Build history of the part. All positions in model axes, mm. Face numbers are marked on the shaded views. Give positions to 0.01 mm unless a question says otherwise; leave off trailing zeros. Loops run counter-clockwise (first coordinate to the right, second up) from the corner with the lowest first, then second, coordinate; pieces in that order, holes last. Notation, with made-up numbers: (15, -6.75) -> (32, -6.75) arc R24 ccw to (32, 20.25) -> close; hole circle Ø10 at (55.25, 40). An arc over 180 degrees is marked (long way). Answer as a JSON object with one key per item and string values. Group by question number.
Q1. Band-saw the part on C-C, the plane x = 7.5. Write the cut outline in (y, z).
Q2. Drop a flat-ended pin along its axis: pin 1 (1.5 mm diameter, centred on x = 18, z = 1, fed in from +Y). Give the stop position or say it passes through.
Q3. Band-saw the part on A-A, the plane y = 0. Write the cut outline in (x, z), plus the area to 3 significant figures.
Q4. Two-plate mould, pull along X, no slides. Class the marked faces 1 and 2: pulls with the +X half, pulls with the -X half, needs draft (parallel to the pull), parting line crosses it, or undercut.
Q5. Band-saw the part on D-D, the plane x = -8.5. Write the cut outline in (y, z).
Q6. Wall check: probe 1 along X at (y, z) = (1.55, -0.7); probe 2 along Y at (x, z) = (-23.5, 0.2); probe 3 along Y at (x, z) = (-2.5, 0.1). Give the ranges that are in metal, low to high. Write a range as from..to.
Autodesk Inventor part; units mm, degrees
ref_plane "YZ Plane" through (0, 0, 0) normal (1, 0, 0) x (0, 1, 0)
ref_plane "XZ Plane" through (0, 0, 0) normal (0, 1, 0) x (-1, 0, 0)
ref_plane "XY Plane" through (0, 0, 0) normal (0, 0, 1) x (1, 0, 0)
sketch "Sketch1" plane through (0, 0, 0) normal (0, 1, 0) x (-1, 0, 0)
  line L0 (13, 2) -> (13, 1.5)
  line L1 (13, 1.5) -> (0, 1.5)
  line L2 (28, 0) -> (28, 2)
  line L3 (28, 2) -> (13, 2)
  line L4 (0, 1.5) -> (0, 2)
  line L5 (0, 2) -> (-30, 2)
  line L6 (-30, 2) -> (-30, 0)
  line L7 (28, 0) -> (0, 0)
  line L8 (0, 0) -> (-30, 0)
  dimension "d5" = 0.5
  dimension "d6" = 15
  dimension "d7" = 0.5
  dimension "d8" = 2
  dimension "d9" = 28
  dimension "d10" = 30
  dimension "d12" = 4
revolve "Revolution1" add sketch "Sketch1" angle 360 about axis through (-28, 0, 0) along (1, 0, 0)
equation "\"d6\" = parA"
equation "\"d9\" = parH"
equation "\"d10\" = stroke"
properties part number "cylinderRod"
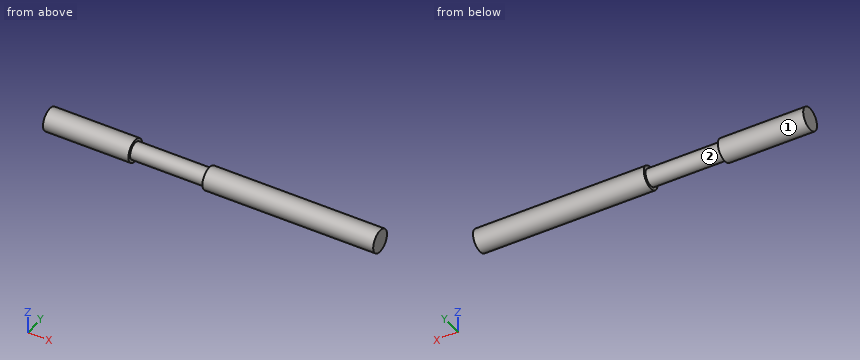
Worked answers:
{
 "1": {"outline": "circle Ø4 at (0, 0)"},
 "2": {"pin 1": "y = 1.98"},
 "3": {"outline": "(-28, -2) -> (-13, -2) -> (-13, -1.5) -> (0, -1.5) -> (0, -2) -> (30, -2) -> (30, 2) -> (0, 2) -> (0, 1.5) -> (-13, 1.5) -> (-13, 2) -> (-28, 2) -> close", "area": "219 mm2"},
 "4": {"face 1": "needs draft", "face 2": "undercut"},
 "5": {"outline": "circle Ø3 at (0, 0)"},
 "6": {"probe 1": "-28..-13, 0..30", "probe 2": "-1.99..1.99", "probe 3": "-1.5..1.5"}
}
